from build123d import *

# Parameters (mm, degrees)
SKETCH_1_W          = 240
SKETCH_1_H          = 65
SKETCH_1_R          = 2.1
SKETCH_1_W_2        = 120
SKETCH_1_H_2        = 15
EXTRUDE_1_DEPTH     = 3
SKETCH_3_R          = 1.6
SKETCH_3_R_2        = 1.55
SKETCH_3_W          = 45
SKETCH_3_H          = 15
CUT_EXTRUDE_2_DEPTH = 254
FILLET_1_R          = 5


with BuildPart() as part:
    # 草图1 → 凸台-拉伸1 (new body)
    # profile 1 of 2: a face of its own
    with BuildSketch(Plane(origin=(0, 0, 0), x_dir=(1, 0, 0), z_dir=(0, 1, 0))):
        with Locations((120, 32.5)):
            Rectangle(SKETCH_1_W, SKETCH_1_H)
        with Locations(Location((225, 20, 0), (0, 0, 270))):
            Circle(SKETCH_1_R, mode=Mode.SUBTRACT)
        with Locations(Location((15, 55, 0), (0, 0, 270))):
            Circle(SKETCH_1_R, mode=Mode.SUBTRACT)
        with Locations(Location((15, 20, 0), (0, 0, 270))):
            Circle(SKETCH_1_R, mode=Mode.SUBTRACT)
        with Locations(Location((225, 55, 0), (0, 0, 270))):
            Circle(SKETCH_1_R, mode=Mode.SUBTRACT)
    # profile 2 of 2: a face of its own
    with BuildSketch(Plane(origin=(0, 0, 0), x_dir=(1, 0, 0), z_dir=(0, 1, 0))):
        with Locations((120, 72.5)):
            Rectangle(SKETCH_1_W_2, SKETCH_1_H_2)
    extrude(amount=EXTRUDE_1_DEPTH)

    # 草图3 → 切除-拉伸2 (cut, through all)
    with BuildSketch(Plane.XZ):
        with Locations(Location((89, -10, 0), (0, 0, 270))):
            Circle(SKETCH_3_R)
        with Locations(Location((151, -10, 0), (0, 0, 90))):
            Circle(SKETCH_3_R)
        with Locations(Location((151, -60, 0), (0, 0, 270))):
            Circle(SKETCH_3_R)
        with Locations(Location((89, -60, 0), (0, 0, 90))):
            Circle(SKETCH_3_R)
        with Locations(Location((106, -3, 0), (0, 0, 270))):
            Circle(SKETCH_3_R_2)
        with Locations(Location((134, -3, 0), (0, 0, 90))):
            Circle(SKETCH_3_R_2)
        with Locations(Location((134, -75, 0), (0, 0, 270))):
            Circle(SKETCH_3_R_2)
        with Locations(Location((106, -75, 0), (0, 0, 90))):
            Circle(SKETCH_3_R_2)
        with Locations((22.5, -7.5)):
            Rectangle(SKETCH_3_W, SKETCH_3_H)
        with Locations((217.5, -7.5)):
            Rectangle(SKETCH_3_W, SKETCH_3_H)
    extrude(amount=-CUT_EXTRUDE_2_DEPTH, mode=Mode.SUBTRACT)

    # 圆角1
    fillet_1_edges = [part.edges().sort_by_distance(p)[0] for p in [
        (0, 1.5, -65),
        (60, 1.5, -65),
        (60, 1.5, -80),
        (180, 1.5, -80),
        (180, 1.5, -65),
        (240, 1.5, -65),
        (45, 1.5, 0),
        (45, 1.5, -15),
        (0, 1.5, -15),
        (240, 1.5, -15),
        (195, 1.5, -15),
        (195, 1.5, 0),
    ]]
    fillet(fillet_1_edges, radius=FILLET_1_R)


solid = part.part
Work out the finished part from the listing and answer in its coordinate system (mm). Round coordinates to 2 decimals unless told otherwise and drop trailing zeros. Write each loop counter-clockwise with the first axis right and the second up, starting at its lowest first coordinate (ties: lowest second). Pieces come first, ordered by that corner, then holes.
1) A cutting plane is placed at A-A (x = 225). Give the vertices of the cut face in (y, z), plus the area to 3 significant figures.
2) The mould has two halves that part along X. Classify faces 1 (the cylindrical face through (1, 2, -63)), 2 (the flat face through (118, 0, -41)), 3 (the cylindrical face through (227.082, 1.479, -55.273)): pulls with the +X half, pulls with the -X half, needs draft (parallel to the pull), parting line crosses it, or undercut.
3) Straight lines are drawn through the part: line 1 (X direction, y = 2.05, z = -20); line 2 (Z direction, x = 151, y = 2.2); line 3 (Z direction, x = 225, y = 2.15). For each, find the intervals that lie inside material, in ascending order.
4) A cutting plane is placed at C-C (y = 2.4). Give the number of separate pieces and of enclosed holes in the cut face, plus the area to 3 significant figures.
5) A cutting plane is placed at B-B (z = -55). Give the vertices of the cut face in (x, y).
6) Given pin 1 Ø1.9 at (x, z) = (106, -3) entering from -Y; pin 2 Ø3.5 at (x, z) = (151, -10) entering from +Y; pin 3 Ø0.9 at (x, y) = (212.5, 1) entering from +Z; pin 4 Ø0.9 at (y, z) = (1.5, -72.5) entering from -X, each flat-ended and moving along its own axis, determine where each tip first touches the part or whether it passes through.
Completed:
1. outline: (0, -65) - (3, -65) - (3, -57.1) - (0, -57.1) - close; (0, -52.9) - (3, -52.9) - (3, -22.1) - (0, -22.1) - close; (0, -17.9) - (3, -17.9) - (3, -15) - (0, -15) - close
1. area: 125 mm2
2. face 1: pulls with the -X half
2. face 2: needs draft
2. face 3: undercut
3. line 1: x = 0 to 12.9, 17.1 to 222.9, 227.1 to 240
3. line 2: z = -80 to -61.6, -58.4 to -11.6, -8.4 to 0
3. line 3: z = -65 to -57.1, -52.9 to -22.1, -17.9 to -15
4. separate pieces: 1
4. enclosed holes: 12
4. area: 15,900 mm2
5. outline: (0, 0) - (12.9, 0) - (12.9, 3) - (0, 3) - close; (17.1, 0) - (222.9, 0) - (222.9, 3) - (17.1, 3) - close; (227.1, 0) - (240, 0) - (240, 3) - (227.1, 3) - close
6. pin 1: passes through
6. pin 2: stops at y = 3
6. pin 3: stops at z = -15
6. pin 4: stops at x = 60
